Can you work these out from the drawing? Everything is in mm from the part's minimum corner. A direction names the side the tool comes from. Coordinates: 2 decimals unless noted, no trailing zeros. Order: outer loops, then holes, each group sorted by start corner. A loop starts at its lowest first (then second) coordinate and runs counter-clockwise, first axis right, second up. Notation, with made-up numbers: (24, 32.25) - (34, 32.25) arc R6 ccw to (34, 41.25) - close; hole circle Ø4 at (83.5, 33). An arc over 180 degrees is marked (long way). Use one line per item in the form item = value. Start each with the question number.
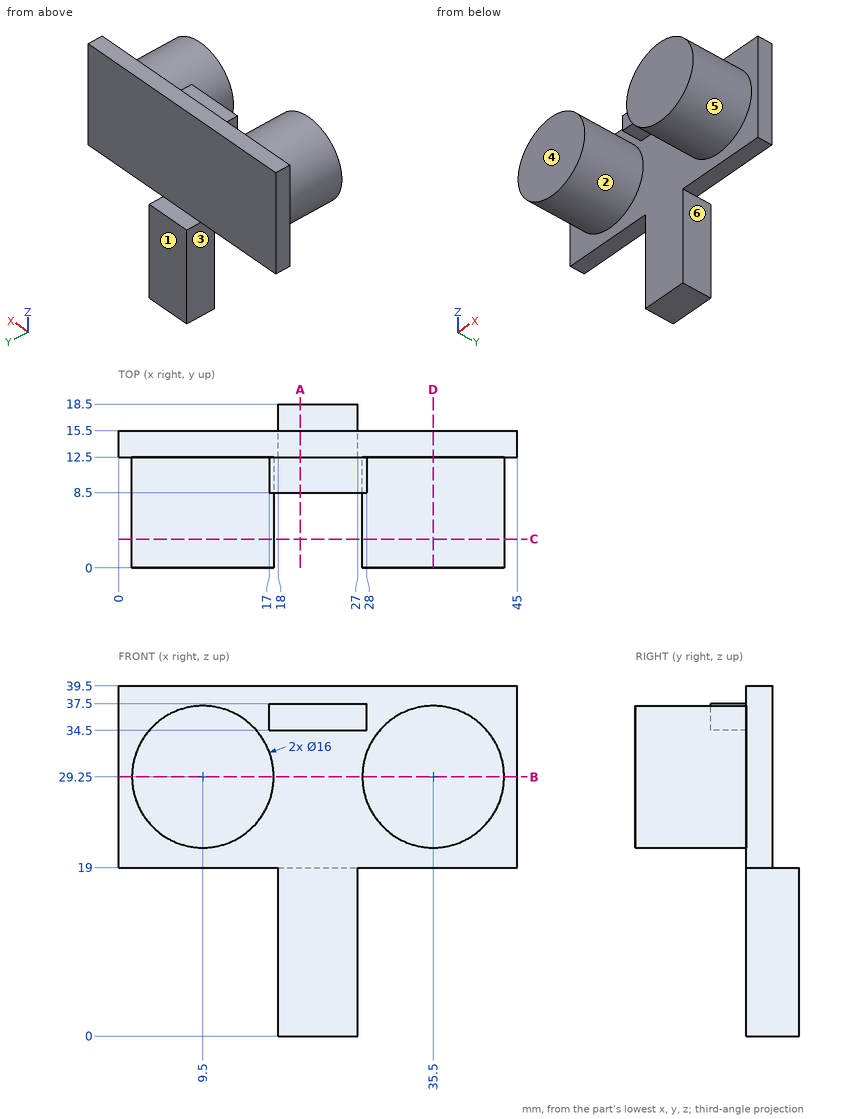
1) If we mould it in two halves opening along X, with no side actions, what happens to the marked faces 4, 5 and 6? For each: pulls with the +X half, pulls with the -X half, needs draft (parallel to the pull), parting line crosses it, or undercut.
2) Suppose I cut it at D-D, the plane x = 35.5. List the corners of the cut face in (y, z) for me.
3) I need wall thicknesses on probe 1 along X at (y, z) = (7.75, 29); probe 2 along Y at (x, z) = (27.5, 37); probe 3 along Z at (x, y) = (33.5, 15.25). Which ranges of each line are inside material? Lowest first, please. Write a range as [from, to].
4) Suppose I cut it at B-B, the plane z = 29.25. List the corners of the cut face in (x, y) for me.
5) For pin 1 (3.5 mm diameter, centred on x = 37.5, y = 14, fed in from -Z); pin 2 (1 mm diameter, centred on x = 11.5, y = 9, fed in from -Z); pin 3 (16.5 mm diameter, centred on x = 24.5, z = 27.5, fed in from +Y), each with a flat end and sliding along its axis, tell me the tip position at first contact or that it passes through.
6) Which directions (+Z, -Z, +X, -X, +Y, -Y) give clear straight access to the entire face, cutting with the end or side of a thin tool? Please do the marked faces 1, 2 and 3.
7) Suppose I cut it at C-C, the plane y = 3.25. List the corners of the cut face in (x, z) for me.
8) Suppose I cut it at A-A, the plane x = 20.5. List the corners of the cut face in (y, z) for me, then the cut area to 4 significant figures.
From the geometry:
q1.face_4 = needs draft
q1.face_5 = undercut
q1.face_6 = pulls with the +X half
q2.outline = (0, 21.25) - (12.5, 21.25) - (12.5, 19) - (15.5, 19) - (15.5, 39.5) - (12.5, 39.5) - (12.5, 37.25) - (0, 37.25) - close
q3.probe_1 = [1.5, 17.5], [27.5, 43.5]
q3.probe_2 = [8.5, 15.5]
q3.probe_3 = [19, 39.5]
q4.outline = (0, 12.5) - (1.5, 12.5) - (1.5, 0) - (17.5, 0) - (17.5, 12.5) - (27.5, 12.5) - (27.5, 0) - (43.5, 0) - (43.5, 12.5) - (45, 12.5) - (45, 15.5) - (0, 15.5) - close
q5.pin_1 = 19
q5.pin_2 = 21.39
q5.pin_3 = 15.5
q6.face_1 = +Z, -Z, +X, -X, +Y
q6.face_2 = -Y
q6.face_3 = -Z, -X, +Y, -Y
q7.outline = circle Ø16 at (9.5, 29.25); circle Ø16 at (35.5, 29.25)
q8.outline = (8.5, 34.5) - (12.5, 34.5) - (12.5, 0) - (18.5, 0) - (18.5, 19) - (15.5, 19) - (15.5, 39.5) - (12.5, 39.5) - (12.5, 37.5) - (8.5, 37.5) - close
q8.area = 187.5 mm2
